```python
from build123d import *

# Parameters (mm, degrees)
SKETCH_1_W      = 220
SKETCH_1_H      = 33
SKETCH_1_R      = 1.5
SKETCH_1_R_2    = 9
SKETCH_1_R_3    = 8
SKETCH_1_R_4    = 1.8
EXTRUDE_1_DEPTH = 3


with BuildPart() as part:
    # 草图1 → 凸台-拉伸1 (new body)
    with BuildSketch(Plane(origin=(0, 0, 0), x_dir=(1, 0, 0), z_dir=(0, 1, 0))):
        with Locations((110, -16.5)):
            Rectangle(SKETCH_1_W, SKETCH_1_H)
        with Locations((5, -27.75)):
            Circle(SKETCH_1_R, mode=Mode.SUBTRACT)
        with Locations((5, -5.45)):
            Circle(SKETCH_1_R, mode=Mode.SUBTRACT)
        with Locations((24.5, -8.7)):
            Circle(SKETCH_1_R, mode=Mode.SUBTRACT)
        with Locations((24.5, -24.3)):
            Circle(SKETCH_1_R, mode=Mode.SUBTRACT)
        with Locations((195.5, -8.7)):
            Circle(SKETCH_1_R, mode=Mode.SUBTRACT)
        with Locations((195.5, -24.3)):
            Circle(SKETCH_1_R, mode=Mode.SUBTRACT)
        with Locations((215, -27.75)):
            Circle(SKETCH_1_R, mode=Mode.SUBTRACT)
        with Locations((215, -5.45)):
            Circle(SKETCH_1_R, mode=Mode.SUBTRACT)
        with Locations((110, -16.5)):
            Circle(SKETCH_1_R_2, mode=Mode.SUBTRACT)
        with Locations((140, -16.5)):
            Circle(SKETCH_1_R_2, mode=Mode.SUBTRACT)
        with Locations((10, -16.5)):
            Circle(SKETCH_1_R_3, mode=Mode.SUBTRACT)
        with Locations((210, -16.5)):
            Circle(SKETCH_1_R_3, mode=Mode.SUBTRACT)
        with Locations((170, -16.5)):
            Circle(SKETCH_1_R_2, mode=Mode.SUBTRACT)
        with Locations((80, -16.5)):
            Circle(SKETCH_1_R_2, mode=Mode.SUBTRACT)
        with Locations((50, -16.5)):
            Circle(SKETCH_1_R_2, mode=Mode.SUBTRACT)
        with Locations((154, -16.5)):
            Circle(SKETCH_1_R_4, mode=Mode.SUBTRACT)
        with Locations((66, -16.5)):
            Circle(SKETCH_1_R_4, mode=Mode.SUBTRACT)
    extrude(amount=EXTRUDE_1_DEPTH)


solid = part.part
```
The listing builds one solid part. Answer for the finished solid, in the listing's coordinates (mm). Round coordinates to 2 decimals unless told otherwise and drop trailing zeros. Write each loop counter-clockwise with the first axis right and the second up, starting at its lowest first coordinate (ties: lowest second). Pieces come first, ordered by that corner, then holes. Notation, with made-up numbers: (68.5, 35.25) -> (104.5, 35.25) arc R8 cw to (104.5, 46.25) -> close; hole circle Ø5 at (23.5, 52.5). An arc over 180 degrees is marked (long way). Write item = value, one per line.
1) Given pin 1 (3 mm diameter, centred on x = 198, z = 7, fed in from -Y), flat-ended and moving along its own axis, determine where the tip first touches the part or whether it passes through.
Check values:
pin_1 = 0
2) Section A-A on x = 140 is taken. Write down the section's boundary in (y, z), plus the area to 3 significant figures.
Check values:
outline = (0, 0) -> (3, 0) -> (3, 7.5) -> (0, 7.5) -> close; (0, 25.5) -> (3, 25.5) -> (3, 33) -> (0, 33) -> close
area = 45.0 mm²
3) For a pull along X with two mould halves and no side action, classify faces 1 (the flat face through (108, 0, 27)), 2 (the cylindrical face through (161.01, 1.48, 16.1)) as released by +X, released by -X, zero draft, split by the parting line, or undercut.
Check values:
face_1 = zero draft
face_2 = undercut
4) Straight lines are drawn through the part: line 1 along X through (y, z) = (0.75, 5.45); line 2 along Z through (x, y) = (195.5, 0.7); line 3 along Z through (x, y) = (210, 1.85). For each, find the intervals that lie inside material, in ascending order. Write a range as [from, to].
Check values:
line_1 = [0, 3.5], [6.5, 213.5], [216.5, 220]
line_2 = [0, 7.2], [10.2, 22.8], [25.8, 33]
line_3 = [0, 8.5], [24.5, 33]
5) Section B-B on y = 0.95 is taken. Give the number of separate pieces and of enclosed holes in the cut face, plus the area to 3 significant figures.
Check values:
separate_pieces = 1
enclosed_holes = 17
area = 5,510 mm²
6) Section C-C on x = 10 is taken. Write down the section's boundary in (y, z), plus the area to 3 significant figures.
Check values:
outline = (0, 0) -> (3, 0) -> (3, 8.5) -> (0, 8.5) -> close; (0, 24.5) -> (3, 24.5) -> (3, 33) -> (0, 33) -> close
area = 51.0 mm²
